from build123d import *

# Parameters (mm, degrees)
SKETCH3_R          = 1.25
CUT_EXTRUDE1_DEPTH = 20.917878903
CUT_EXTRUDE2_DEPTH = 5
SKETCH4_R          = 1.175
CUT_EXTRUDE3_DEPTH = 20.601579018
CHAMFER1_SIZE      = 0.5
FILLET1_R          = 1


with BuildPart() as part:
    # Sketch2 → Revolve2 (revolve)
    with BuildSketch(Plane.XY):
        Polygon((4.1, 0), (10.25, 0), (10.25, 5), (12.87, 6.09), (12.87, 8.09), (4.1, 8.09), align=None)
    revolve(axis=Axis((0, 8.09, 0), (0, -1, 0)))

    # Sketch3 → Cut-Extrude1 (cut, through all)
    with BuildSketch(Plane.XZ):
        with Locations(Location((0, 8, 0), (0, 0, 270))):
            Circle(SKETCH3_R)
        with Locations(Location((8, 0, 0), (0, 0, 270))):
            Circle(SKETCH3_R)
        with Locations(Location((0, -8, 0), (0, 0, 270))):
            Circle(SKETCH3_R)
        with Locations(Location((-8, 0, 0), (0, 0, 270))):
            Circle(SKETCH3_R)
    extrude(amount=-CUT_EXTRUDE1_DEPTH, mode=Mode.SUBTRACT)

    # Sketch5 → Cut-Extrude2 (cut)
    with BuildSketch(Plane(origin=(0, 8.09, 0), x_dir=(1, 0, 0), z_dir=(0, 1, 0))):
        with BuildLine():
            Line((-2.5, -8), (-2.5, -14))
            Line((-2.5, -14), (2.5, -14))
            Line((2.5, -14), (2.5, -8))
            ThreePointArc((2.5, -8), (0, -5.5), (-2.5, -8))
        make_face()
        with BuildLine():
            Line((-8, 2.5), (-14, 2.5))
            Line((-14, 2.5), (-14, -2.5))
            Line((-14, -2.5), (-8, -2.5))
            ThreePointArc((-8, -2.5), (-5.5, 0), (-8, 2.5))
        make_face()
        with BuildLine():
            Line((2.5, 8), (2.5, 14))
            Line((2.5, 14), (-2.5, 14))
            Line((-2.5, 14), (-2.5, 8))
            ThreePointArc((-2.5, 8), (0, 5.5), (2.5, 8))
        make_face()
        with BuildLine():
            Line((8, -2.5), (14, -2.5))
            Line((14, -2.5), (14, 2.5))
            Line((14, 2.5), (8, 2.5))
            ThreePointArc((8, 2.5), (5.5, 0), (8, -2.5))
        make_face()
    extrude(amount=-CUT_EXTRUDE2_DEPTH, mode=Mode.SUBTRACT)

    # Sketch4 → Cut-Extrude3 (cut, through all)
    with BuildSketch(Plane(origin=(0, 8.09, 0), x_dir=(1, 0, 0), z_dir=(0, 1, 0))):
        with Locations(Location((-7.336232855, 7.336232855, 0), (0, 0, 270))):
            Circle(SKETCH4_R)
        with Locations(Location((7.336232855, -7.336232855, 0), (0, 0, 270))):
            Circle(SKETCH4_R)
    extrude(amount=-CUT_EXTRUDE3_DEPTH, mode=Mode.SUBTRACT)

    # Chamfer1
    chamfer1_edges = [part.edges().sort_by_distance(p)[0] for p in [
        (7.336232855, 8.09, 6.161232855),
        (-7.336232855, 8.09, -8.511232855),
    ]]
    chamfer(chamfer1_edges, length=CHAMFER1_SIZE)

    # Fillet1
    fillet1_edges = [part.edges().sort_by_distance(p)[0] for p in [
        (-2.5, 7.09, -12.624852474),
        (2.5, 7.09, -12.624852474),
        (-12.624852474, 7.09, 2.5),
        (-12.624852474, 7.09, -2.5),
        (12.624852474, 7.09, -2.5),
        (12.624852474, 7.09, 2.5),
        (2.5, 7.09, 12.624852474),
        (-2.5, 7.09, 12.624852474),
    ]]
    fillet(fillet1_edges, radius=FILLET1_R)


solid = part.part
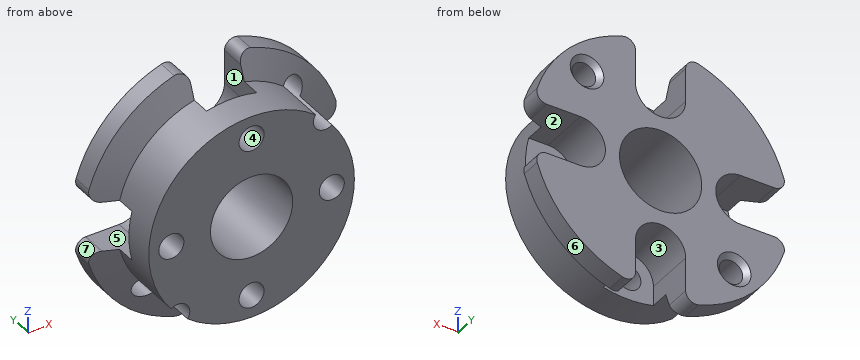
Here's how the part is built. I have some questions about the finished solid (model axes, mm). Face numbers are marked on the shaded views. A direction names the side the tool comes from. Coordinates: 2 decimals unless noted, no trailing zeros. Order: outer loops, then holes, each group sorted by start corner. A loop starts at its lowest first (then second) coordinate and runs counter-clockwise, first axis right, second up. Notation, with made-up numbers: M -12.5,35.5 L 41.5,35.5 A9 ccw 41.5,46.5 Z; hole C -4.75,53.25 d7. An arc over 180 degrees is marked long. Answer as CSV lines item,"result". Start each with the question number.
1. I want a section at C-C, the plane y = 1.25. Count the separate pieces of the cut face and the enclosed holes in it, and give its area (3 significant figures).
2. I need wall thicknesses on line 1 (Z direction, x = 0.5, y = 2.25); line 2 (Z direction, x = -3.25, y = 7.5); line 3 (Z direction, x = -2.25, y = 2.75). Which ranges of each line are inside material? Lowest first, please. Write a range as [from, to].
3. We'd pull the mould along X, two halves only. Please class the marked faces 4, 5, 6 and 7: released by +X, released by -X, zero draft, split by the parting line, or undercut.
4. For pin 1 (2.5 mm diameter, centred on x = -9, y = 5, fed in from -Z); pin 2 (4 mm diameter, centred on y = 5.5, z = -9, fed in from -X); pin 3 (3.5 mm diameter, centred on y = 4.5, z = 9, fed in from -X); pin 4 (6.5 mm diameter, centred on x = 0, z = 0, fed in from -Y), each with a flat end and sliding along its axis, tell me the tip position at first contact or that it passes through.
5. I want a section at B-B, the plane y = 7. Write out the boundary of the cut face in (x, z) (3 decimals).
6. On a 3-axis mill with a long thin cutter (end or side, diameter ignored), from which of +Z, -Z, +X, -X, +Y, -Y can I reach the whole of each face in a straight line? I mean the marked faces 1, 2 and 3. Say none if no direction works.
7. I want a section at A-A, the plane z = 0. Write out the boundary of the cut face in (x, y).
Recorded:
1,separate pieces,"1"
1,enclosed holes,"5"
1,area,"254 mm2"
2,line 1,"z = [-10.24, -9.15], [-6.85, -4.07], [4.07, 6.85], [9.15, 10.24]"
2,line 2,"z = [-12.31, -2.5], [2.5, 12.31]"
2,line 3,"z = [-10, -3.43], [3.43, 10]"
3,face 4,"undercut"
3,face 5,"zero draft"
3,face 6,"released by +X"
3,face 7,"released by -X"
4,pin 1,"stops at z = -9.76"
4,pin 2,"stops at x = -10.74"
4,pin 3,"stops at x = -9.86"
4,pin 4,"passes through"
5,outline,"M -12.298,-3.795 A12.87 ccw -3.795,-12.298 A1 ccw -2.5,-11.342 L -2.5,-8 A2.5 cw 2.5,-8 L 2.5,-11.342 A1 ccw 3.795,-12.298 A12.87 ccw 12.298,-3.795 A1 ccw 11.342,-2.5 L 8,-2.5 A2.5 cw 8,2.5 L 11.342,2.5 A1 ccw 12.298,3.795 A12.87 ccw 3.795,12.298 A1 ccw 2.5,11.342 L 2.5,8 A2.5 cw -2.5,8 L -2.5,11.342 A1 ccw -3.795,12.298 A12.87 ccw -12.298,3.795 A1 ccw -11.342,2.5 L -8,2.5 A2.5 cw -8,-2.5 L -11.342,-2.5 A1 ccw Z; hole C -7.336,-7.336 d2.35; hole C 0,0 d8.2; hole C 7.336,7.336 d2.35"
6,face 1,"+Z, +Y"
6,face 2,"+X, +Y"
6,face 3,"-Z, +Y"
7,outline,"M -10.25,0 L -9.25,0 L -9.25,3.09 L -10.25,3.09 Z; M -6.75,0 L -4.1,0 L -4.1,8.09 L -5.5,8.09 L -5.5,3.09 L -6.75,3.09 Z; M 4.1,0 L 6.75,0 L 6.75,3.09 L 5.5,3.09 L 5.5,8.09 L 4.1,8.09 Z; M 9.25,0 L 10.25,0 L 10.25,3.09 L 9.25,3.09 Z"
